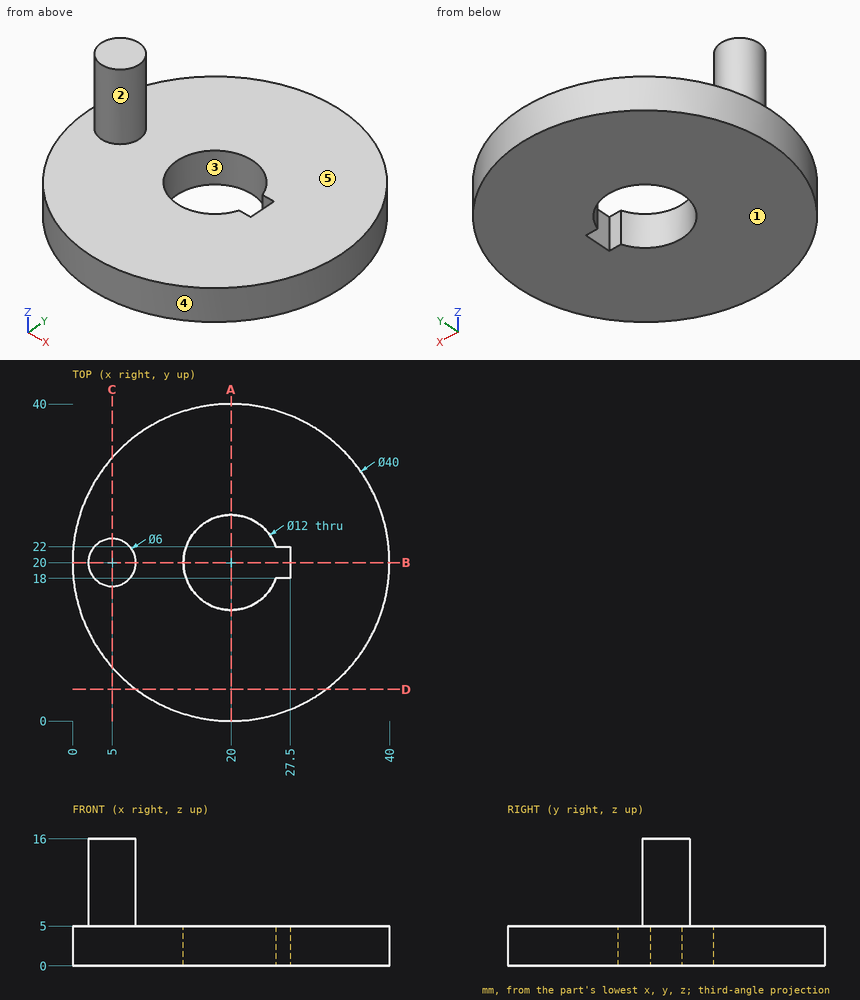
Geometry check sheet. Reference: drawing and pictorial views, mm from the part's lowest x, y, z. A direction names the side the tool comes from. Coordinates: 2 decimals unless noted, no trailing zeros. Write each loop counter-clockwise with the first axis right and the second up, starting at its lowest first coordinate (ties: lowest second). Pieces come first, ordered by that corner, then holes.
Item 1: Access from +Z, -Z, +X, -X, +Y, -Y to the whole of each face (thin tool, end or side, straight path). Record for the marked faces 1 and 2.
Numbers:
face 1: -Z, +X, -X, +Y, -Y
face 2: +Z
Item 2: Scan lines: probe 1 along Y at (x, z) = (20, 1.65); probe 2 along Z at (x, y) = (26, 8); probe 3 along X at (y, z) = (22, 5.5). Record each from-to range of solid material in increasing order.
Numbers:
probe 1: y = 0 to 14, 26 to 40
probe 2: z = 0 to 5
probe 3: x = 2.76 to 7.24
Item 3: Depth check by flat-ended pin: pin 1 Ø3 at (y, z) = (13.5, 4.5) entering from -X; pin 2 Ø1.5 at (y, z) = (19, 11.5) entering from +X; pin 3 Ø5 at (y, z) = (30.5, 3.5) entering from -X. Enter the tip coordinate at first touch or a pass-through.
Numbers:
pin 1: stops at x = 0.64
pin 2: stops at x = 7.99
pin 3: stops at x = 1.67
Item 4: Cross-section at C-C on x = 5. Record the boundary of the cut face in (y, z), then the cut area to 3 significant figures.
Numbers:
outline: (6.77, 0) - (33.23, 0) - (33.23, 5) - (23, 5) - (23, 16) - (17, 16) - (17, 5) - (6.77, 5) - close
area: 198 mm2
Item 5: Cross-section at D-D on y = 4. Record the boundary of the cut face in (x, z), then the cut area to 3 significant figures.
Numbers:
outline: (8, 0) - (32, 0) - (32, 5) - (8, 5) - close
area: 120 mm2
Item 6: Cross-section at B-B on y = 20. Record the boundary of the cut face in (x, z), then the cut area to 4 significant figures.
Numbers:
outline: (0, 0) - (14, 0) - (14, 5) - (8, 5) - (8, 16) - (2, 16) - (2, 5) - (0, 5) - close; (27.5, 0) - (40, 0) - (40, 5) - (27.5, 5) - close
area: 198.5 mm2
Item 7: Cross-section at A-A on x = 20. Record the boundary of the cut face in (y, z).
Numbers:
outline: (0, 0) - (14, 0) - (14, 5) - (0, 5) - close; (26, 0) - (40, 0) - (40, 5) - (26, 5) - close
Item 8: Mould release check, pull along Y, two halves, no side actions. Record for the marked faces 3, 4 and 5: released by +Y, released by -Y, zero draft, split by the parting line, or undercut.
Numbers:
face 3: undercut
face 4: split by the parting line
face 5: zero draft
